For this review, use the dimensioned drawing (mm, ordinates from the lowest corner) and the shaded views. Round coordinates to 2 decimals unless told otherwise and drop trailing zeros. Loops run counter-clockwise (first coordinate to the right, second up) from the corner with the lowest first, then second, coordinate; pieces in that order, holes last. Notation, with made-up numbers: (87, 11) - (101, 11) arc R28 cw to (101, 48) - close; hole circle Ø11 at (38.5, 5). An arc over 180 degrees is marked (long way). One line per question, with ' | ' between items. Start each with the question number.
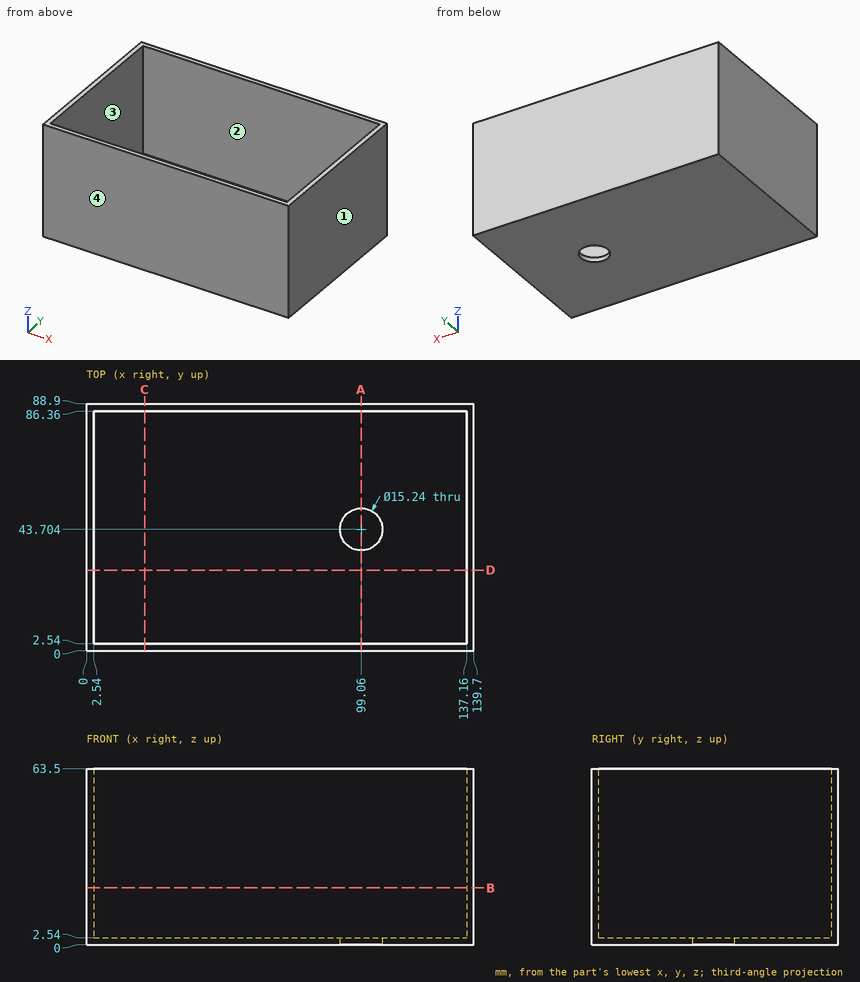
1. To check wall thickness, follow line 1 along Y through (x, z) = (99, 1); line 2 along Y through (x, z) = (110, 12); line 3 along X through (y, z) = (28, 4). State the ranges of each line that lie inside material, in increasing order.
2. Take a section at D-D, the plane y = 29. Give the boundary of the cut face in (x, z).
3. Clearance check with a flat-ended pin moving along its axis: P1, Ø1, axis at x = 86.5, y = 45.5, coming from the +Z side. State where the tip first meets the part, or that it passes through.
4. Take a section at B-B, the plane z = 20.5. Give the boundary of the cut face in (x, y), then the cut area to 3 significant figures.
5. The part is to be moulded in two halves that separate along X. For the marked faces 1, 2, 3 and 4, say which applies: pulls with the +X half, pulls with the -X half, needs draft (parallel to the pull), parting line crosses it, or undercut.
6. Take a section at C-C, the plane x = 21. Give the boundary of the cut face in (y, z).
7. Take a section at A-A, the plane x = 99.06. Give the boundary of the cut face in (y, z), then the cut area to 3 significant figures.
Answer list:
1) line 1: y = 0 to 36.08, 51.32 to 88.9 | line 2: y = 0 to 2.54, 86.36 to 88.9 | line 3: x = 0 to 2.54, 137.16 to 139.7
2) outline: (0, 0) - (139.7, 0) - (139.7, 63.5) - (137.16, 63.5) - (137.16, 2.54) - (2.54, 2.54) - (2.54, 63.5) - (0, 63.5) - close
3) P1: stops at z = 2.54
4) outline: (0, 0) - (139.7, 0) - (139.7, 88.9) - (0, 88.9) - close; hole (2.54, 2.54) - (137.16, 2.54) - (137.16, 86.36) - (2.54, 86.36) - close | area: 1,140 mm²
5) face 1: pulls with the +X half | face 2: undercut | face 3: undercut | face 4: needs draft
6) outline: (0, 0) - (88.9, 0) - (88.9, 63.5) - (86.36, 63.5) - (86.36, 2.54) - (2.54, 2.54) - (2.54, 63.5) - (0, 63.5) - close
7) outline: (0, 0) - (36.08, 0) - (36.08, 2.54) - (2.54, 2.54) - (2.54, 63.5) - (0, 63.5) - close; (51.32, 0) - (88.9, 0) - (88.9, 63.5) - (86.36, 63.5) - (86.36, 2.54) - (51.32, 2.54) - close | area: 497 mm²
